Geometry: see drawing. Coordinates: mm, zero at the bounding-box minimum. A direction names the side the tool comes from. Round coordinates to 2 decimals unless told otherwise and drop trailing zeros. Write each loop counter-clockwise with the first axis right and the second up, starting at its lowest first coordinate (ties: lowest second). Pieces come first, ordered by that corner, then holes.
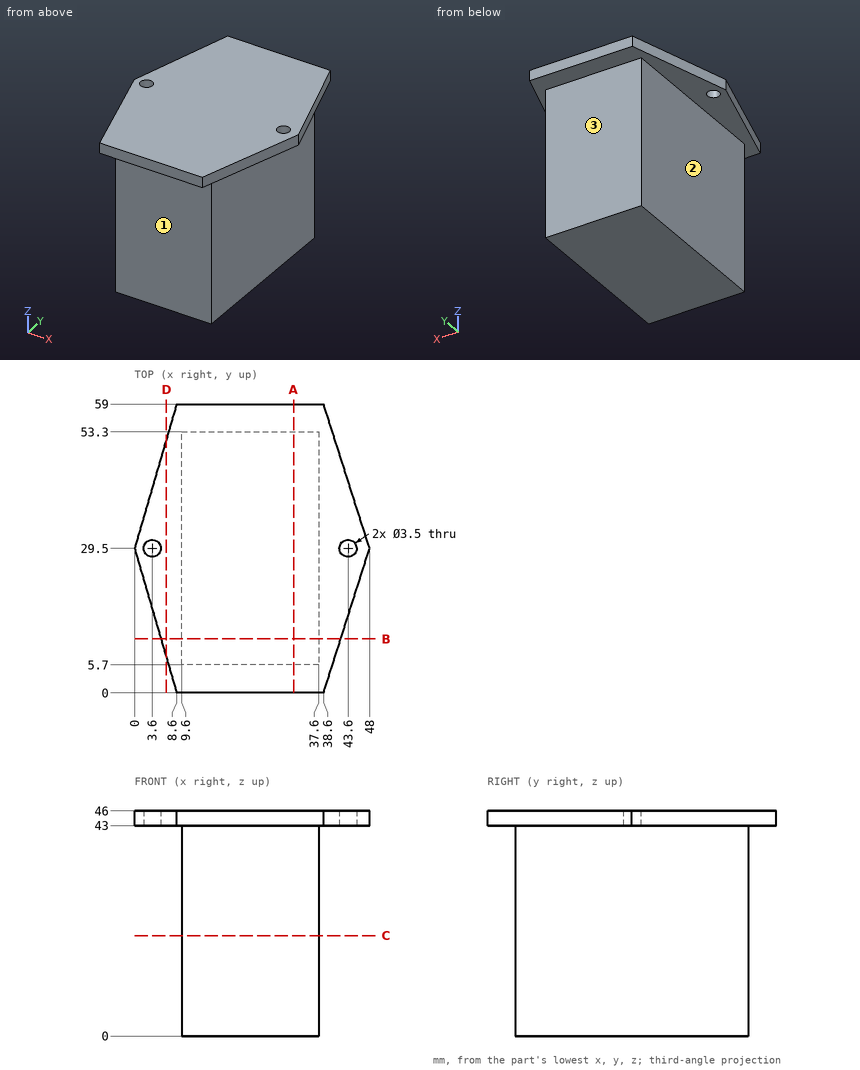
1) Section query A-A on x = 32.5. Return the cut outline in (y, z).
Taken from the geometry:
outline: (0, 43) - (5.7, 43) - (5.7, 0) - (53.3, 0) - (53.3, 43) - (59, 43) - (59, 46) - (0, 46) - close
2) Section query C-C on z = 20.5. Return the cut outline in (x, y), then the cut area to 3 significant figures.
Taken from the geometry:
outline: (9.6, 5.7) - (37.6, 5.7) - (37.6, 53.3) - (9.6, 53.3) - close
area: 1,330 mm2
3) Material intervals for line 1 (X direction, y = 29, z = 44) (1 decimal); line 2 (X direction, y = 28.5, z = 6.5); line 3 (Z direction, x = 17, y = 56), sorted ascending.
Taken from the geometry:
line 1: x = 0.1 to 1.9, 5.3 to 41.9, 45.3 to 47.8
line 2: x = 9.6 to 37.6
line 3: z = 43 to 46
4) Contact query for flat-ended pins moving along their axis: P1, Ø1, axis at y = 9.5, z = 28, coming from the +X side; P2, Ø8.5, axis at x = 24.5, z = 16, coming from the +Y side; P3, Ø8.5, axis at x = 19, z = 31.5, coming from the -Y side; P4, Ø3, axis at x = 3.6, y = 29.5, coming from the -Z side. Output: stop coordinate, or through.
Taken from the geometry:
P1: stops at x = 37.6
P2: stops at y = 53.3
P3: stops at y = 5.7
P4: passes through
5) Reachability of the marked faces 1, 2 and 3 from +Z, -Z, +X, -X, +Y, -Y: full face, straight path, thin tool, end or side. Return the list, or none.
Taken from the geometry:
face 1: -Z, +X, -X, -Y
face 2: -Z, -X, +Y, -Y
face 3: -Z, +X, -X, +Y
6) Section query B-B on y = 11. Return the cut outline in (x, z) (1 decimal), then the cut area to 3 significant figures.
Taken from the geometry:
outline: (5.4, 43) - (9.6, 43) - (9.6, 0) - (37.6, 0) - (37.6, 43) - (42.1, 43) - (42.1, 46) - (5.4, 46) - close
area: 1,310 mm2
7) Section query D-D on x = 6.5. Return the cut outline in (y, z), then the cut area to 3 significant figures.
Taken from the geometry:
outline: (7.2, 43) - (51.8, 43) - (51.8, 46) - (7.2, 46) - close
area: 134 mm2
